Source: three-view drawing plus pictorial views. Frame: mm from the lowest corner of the part. A direction names the side the tool comes from. Give positions to 0.01 mm unless a question says otherwise; leave off trailing zeros. Loops run counter-clockwise (first coordinate to the right, second up) from the corner with the lowest first, then second, coordinate; pieces in that order, holes last. Notation, with made-up numbers: (44.5, 24.5) - (74.5, 24.5) arc R32 ccw to (74.5, 56.5) - close; hole circle Ø11 at (-4.5, -32). An arc over 180 degrees is marked (long way). Answer as a JSON object with one key per item and string values.
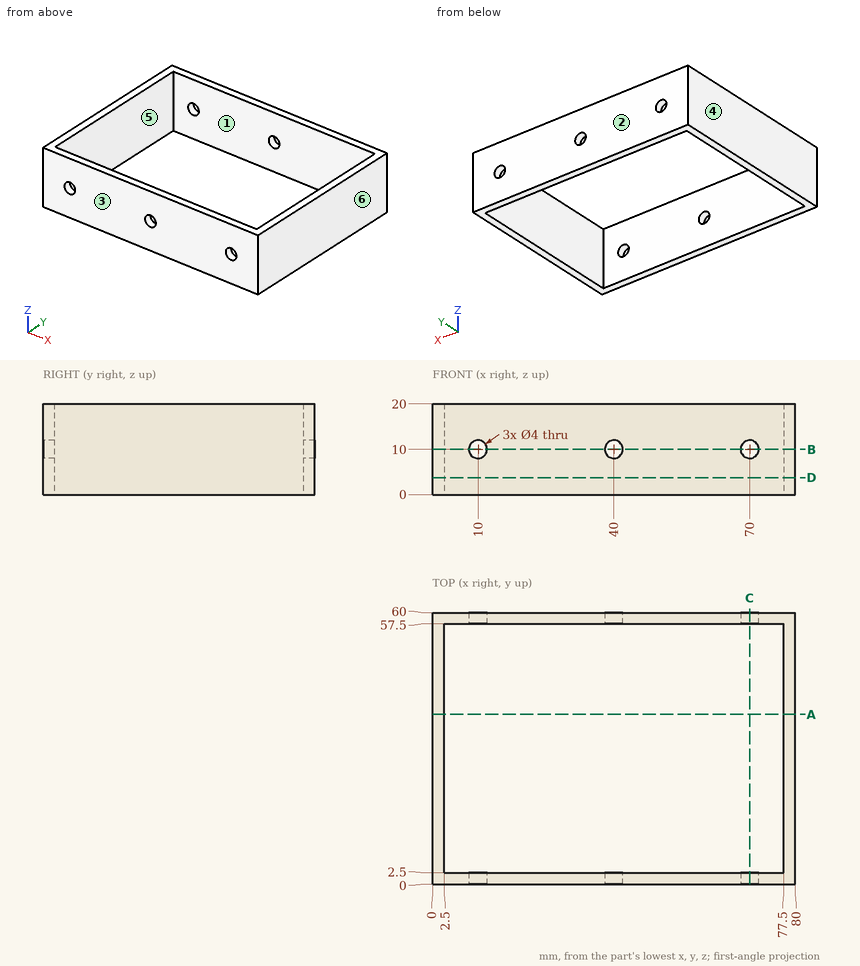
Item 1: Contact query for a flat-ended pin moving along its axis: P1, Ø3, axis at x = 40, z = 10, coming from the +Y side. Output: stop coordinate, or through.
Geometry check:
{"P1": "passes through"}
Item 2: Access query for the marked faces 5 and 6. Directions: +Z, -Z, +X, -X, +Y, -Y. A direction counts if a zero-diameter tool reaches every point of the face in a straight line with its end or side. Return the directions, or none.
Geometry check:
{"face 5": "+Z, -Z", "face 6": "+Z, -Z, +X, +Y, -Y"}
Item 3: Cut plane C-C (x = 70). Return loops of the section in (y, z), then the cut area to 3 significant figures.
Geometry check:
{"outline": "(0, 0) - (2.5, 0) - (2.5, 8) - (0, 8) - close; (0, 12) - (2.5, 12) - (2.5, 20) - (0, 20) - close; (57.5, 0) - (60, 0) - (60, 8) - (57.5, 8) - close; (57.5, 12) - (60, 12) - (60, 20) - (57.5, 20) - close", "area": "80.0 mm2"}
Item 4: Mould query, pull axis Y, two halves, no side actions, for the marked faces 1, 2, 3 and 4. Classes: released by +Y, released by -Y, zero draft, split by the parting line, or undercut.
Geometry check:
{"face 1": "undercut", "face 2": "released by +Y", "face 3": "released by -Y", "face 4": "zero draft"}
Item 5: Cut plane A-A (y = 37.5). Return loops of the section in (x, z), then the cut area to 3 significant figures.
Geometry check:
{"outline": "(0, 0) - (2.5, 0) - (2.5, 20) - (0, 20) - close; (77.5, 0) - (80, 0) - (80, 20) - (77.5, 20) - close", "area": "100 mm2"}
Item 6: Cut plane D-D (z = 3.75). Return loops of the section in (x, y), then the cut area to 3 significant figures.
Geometry check:
{"outline": "(0, 0) - (80, 0) - (80, 60) - (0, 60) - close; hole (2.5, 2.5) - (77.5, 2.5) - (77.5, 57.5) - (2.5, 57.5) - close", "area": "675 mm2"}
Item 7: Material intervals for line 1 (Y direction, x = 8, z = 1.75); line 2 (X direction, y = 42.5, z = 9); line 3 (Z direction, x = 70, y = 59), sorted ascending. Write a range as [from, to].
Geometry check:
{"line 1": "y = [0, 2.5], [57.5, 60]", "line 2": "x = [0, 2.5], [77.5, 80]", "line 3": "z = [0, 8], [12, 20]"}
Item 8: Cut plane B-B (z = 10). Give the number of separate pieces and of enclosed holes in the cut face, then the cut area to 3 significant figures.
Geometry check:
{"separate pieces": "6", "enclosed holes": "0", "area": "615 mm2"}
